Model file for the job. Use its own axes, mm. A direction names the side the tool comes from. Coordinates: 2 decimals unless noted, no trailing zeros. Loops run counter-clockwise (first coordinate to the right, second up) from the corner with the lowest first, then second, coordinate; pieces in that order, holes last.
from build123d import *

# Parameters (mm, degrees)
ESQUISSE1_W             = 7
ESQUISSE1_H             = 5.5
BOSS_EXTRU_1_DEPTH      = 6
BOSS_EXTRU_2_DEPTH      = 0.5
BOSS_EXTRU_2_DEPTH_BACK = 7.5
ESQUISSE2_W             = 5.5
ESQUISSE2_H             = 5.5
ENL_V_MAT_EXTRU_2_DEPTH = 3
ESQUISSE4_W             = 1.5
ESQUISSE4_H             = 1
ESQUISSE4_W_2           = 1
ESQUISSE4_H_2           = 1.5
BOSS_EXTRU_3_DEPTH      = 4
ESQUISSE5_R             = 2
ENL_V_MAT_EXTRU_3_DEPTH = 2
ESQUISSE6_R             = 1
BOSS_EXTRU_4_DEPTH      = 8
CHANFREIN1_SIZE         = 0.5


with BuildPart() as part:
    # Esquisse1 → Boss.-Extru.1 (new body)
    with BuildSketch(Plane(origin=(0, 0, 0), x_dir=(1, 0, 0), z_dir=(0, 1, 0))):
        Rectangle(ESQUISSE1_W, ESQUISSE1_H)
    extrude(amount=BOSS_EXTRU_1_DEPTH)

    # Esquisse3 → Boss.-Extru.2 (add, two sides: drawn at the far end of the back side and taken through both)
    with BuildSketch(Plane.ZY.offset(3.5).offset(-BOSS_EXTRU_2_DEPTH_BACK)):
        Polygon((0, 0), (-1, 0), (-1, 4), (-0.5, 4), (-0.5, 5), (0.5, 5), (0.5, 4), (1, 4), (1, 0), align=None)
    extrude(amount=BOSS_EXTRU_2_DEPTH + BOSS_EXTRU_2_DEPTH_BACK)

    # Esquisse2 → Enlèv. mat.-Extru.2 (cut)
    with BuildSketch(Plane.XZ):
        Rectangle(ESQUISSE2_W, ESQUISSE2_H)
    extrude(amount=-ENL_V_MAT_EXTRU_2_DEPTH, mode=Mode.SUBTRACT)

    # Esquisse4 → Boss.-Extru.3 (add)
    with BuildSketch(Plane(origin=(0, 6, 0), x_dir=(1, 0, 0), z_dir=(0, 1, 0))):
        with Locations((1.25, 0)):
            Rectangle(ESQUISSE4_W, ESQUISSE4_H)
        with Locations((0, -1.25)):
            Rectangle(ESQUISSE4_W_2, ESQUISSE4_H_2)
        with Locations((-1.25, 0)):
            Rectangle(ESQUISSE4_W, ESQUISSE4_H)
        Rectangle(ESQUISSE4_W_2, ESQUISSE4_H)
        with Locations((0, 1.25)):
            Rectangle(ESQUISSE4_W_2, ESQUISSE4_H_2)
    extrude(amount=BOSS_EXTRU_3_DEPTH)

    # Esquisse5 → Enlèv. mat.-Extru.3 (cut)
    with BuildSketch(Plane.XZ.offset(-3)):
        with Locations(Location((0, 0, 0), (0, 0, 270))):
            Circle(ESQUISSE5_R)
    extrude(amount=-ENL_V_MAT_EXTRU_3_DEPTH, mode=Mode.SUBTRACT)

    # Esquisse6 → Boss.-Extru.4 (add)
    with BuildSketch(Plane.XZ.offset(-5)):
        with Locations(Location((0, 0, 0), (0, 0, 270))):
            Circle(ESQUISSE6_R)
    extrude(amount=BOSS_EXTRU_4_DEPTH)

    # Chanfrein1
    chanfrein1_edges = [part.edges().sort_by_distance(p)[0] for p in [
        (0, -3, 1),
        (-3.5, 6, 0),
        (0, 6, 2.75),
        (3.5, 6, 0),
        (0, 6, -2.75),
    ]]
    chamfer(chanfrein1_edges, length=CHANFREIN1_SIZE)


solid = part.part
Q1. Drill centre lines: line 1 (X direction, y = 3.4, z = 0); line 2 (X direction, y = 6.5, z = 0.75); line 3 (Y direction, x = -1.25, z = 1.9). Where is each one in solid material? Low to high.
Answers:
line 1: x = -4 to -2, -1 to 1, 2 to 4
line 2: x = -0.5 to 0.5
line 3: y = 3 to 6
Q2. Which spindle directions (+Z, -Z, +X, -X, +Y, -Y) get a long thin tool onto all of the face, cutting with end or side? Do faces 1 (the flat face through (-2, 8, 0)), 2 (the flat face through (1, 8, -0.5)), 3 (the flat face through (2.75, 1, 0)), 4 (the flat face through (3, 0, 0)), 5 (the flat face through (-0.5, 8, -1)). Say none if no direction does.
Answers:
face 1: +Z, -Z, -X, +Y
face 2: -Z, +X, +Y
face 3: +Z, -Z, -Y
face 4: +Z, -Z, +X, -Y
face 5: -Z, -X, +Y
Q3. Flat gauge pins, fed straight in: P1, Ø1.2, axis at x = -1.5, y = 8.5, coming from the -Z side; P2, Ø1.2, axis at y = 8, z = 1, coming from the +X side; P3, Ø1.6, axis at x = 1, y = 7.5, coming from the -Z side. Where does each tip first touch, or does it go through?
Answers:
P1: stops at z = -0.5
P2: stops at x = 2
P3: stops at z = -2
Q4. Slice it at C-C (x = 0). List the corners of the cut face in (y, z), and give its area (3 significant figures).
Answers:
outline: (-3, -0.5) - (-2.5, -1) - (5, -1) - (5, -2) - (3, -2) - (3, -2.75) - (5.5, -2.75) - (6, -2.25) - (6, -2) - (10, -2) - (10, 2) - (6, 2) - (6, 2.25) - (5.5, 2.75) - (3, 2.75) - (3, 2) - (5, 2) - (5, 1) - (-2.5, 1) - (-3, 0.5) - close
area: 40.0 mm2
Q5. Slice it at A-A (y = 0.25). List the corners of the cut face in (x, z), and give its area (3 significant figures).
Answers:
outline: (-4, -1) - (-3.5, -1) - (-3.5, -2.75) - (-2.75, -2.75) - (-2.75, 2.75) - (-3.5, 2.75) - (-3.5, 1) - (-4, 1) - close; circle Ø2 at (0, 0); (2.75, -2.75) - (3.5, -2.75) - (3.5, -1) - (4, -1) - (4, 1) - (3.5, 1) - (3.5, 2.75) - (2.75, 2.75) - close
area: 13.4 mm2
Q6. Slice it at B-B (z = 0). List the corners of the cut face in (x, y).
Answers:
outline: (-4, 0) - (-2.75, 0) - (-2.75, 3) - (-2, 3) - (-2, 5) - (-1, 5) - (-1, -2.5) - (-0.5, -3) - (0.5, -3) - (1, -2.5) - (1, 5) - (2, 5) - (2, 3) - (2.75, 3) - (2.75, 0) - (4, 0) - (4, 5) - (3.5, 5) - (3.5, 5.5) - (3, 6) - (2, 6) - (2, 10) - (-2, 10) - (-2, 6) - (-3, 6) - (-3.5, 5.5) - (-3.5, 5) - (-4, 5) - close
Q7. Slice it at D-D (y = 8). List the corners of the cut face in (x, z).
Answers:
outline: (-2, -0.5) - (-0.5, -0.5) - (-0.5, -2) - (0.5, -2) - (0.5, -0.5) - (2, -0.5) - (2, 0.5) - (0.5, 0.5) - (0.5, 2) - (-0.5, 2) - (-0.5, 0.5) - (-2, 0.5) - close
